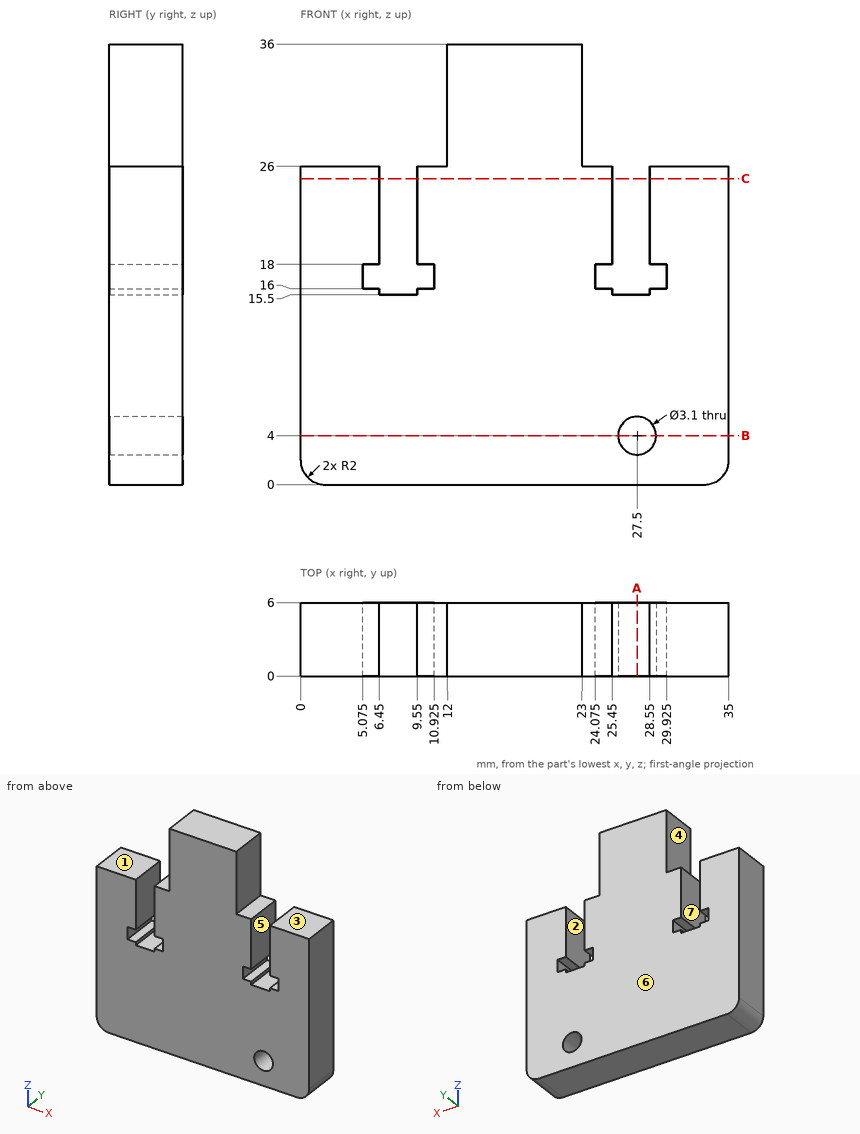
Input: dimensioned drawing with shaded views. Units: mm. Origin: part minimum x, y, z. A direction names the side the tool comes from. Round coordinates to 2 decimals unless told otherwise and drop trailing zeros. Loops run counter-clockwise (first coordinate to the right, second up) from the corner with the lowest first, then second, coordinate; pieces in that order, holes last.
1) Set-up query: the marked faces 1, 2 and 3. Return all of +Z, -Z, +X, -X, +Y, -Y with unobstructed straight access to the full face (end or side cutting, diameter ignored); none if empty.
Ans:
face 1: +Z, -X, +Y, -Y
face 2: +Z, +Y, -Y
face 3: +Z, +X, +Y, -Y
2) Section query C-C on z = 25. Return the cut outline in (x, y), plus the area to 3 significant figures.
Ans:
outline: (0, 0) - (6.45, 0) - (6.45, 6) - (0, 6) - close; (9.55, 0) - (25.45, 0) - (25.45, 6) - (9.55, 6) - close; (28.55, 0) - (35, 0) - (35, 6) - (28.55, 6) - close
area: 173 mm2
3) Pin query (flat end, axial travel): pin 1 (1.8 mm diameter, centred on y = 2, z = 30, fed in from -X); pin 2 (1.5 mm diameter, centred on x = 27, y = 3, fed in from +Z); pin 3 (0.7 mm diameter, centred on x = 23.5, y = 3, fed in from +Z). Return the tip coordinate at first contact, or that it passes through.
Ans:
pin 1: stops at x = 12
pin 2: stops at z = 15.5
pin 3: stops at z = 26
4) Pull-direction query (X, two-part tool) for the marked faces 4, 5, 6 and 7; classes: released by +X, released by -X, zero draft, split by the parting line, or undercut.
Ans:
face 4: released by -X
face 5: undercut
face 6: zero draft
face 7: undercut
5) Section query A-A on x = 27.5. Return the cut outline in (y, z), plus the area to 3 significant figures.
Ans:
outline: (0, 0) - (6, 0) - (6, 2.45) - (0, 2.45) - close; (0, 5.55) - (6, 5.55) - (6, 15.5) - (0, 15.5) - close
area: 74.4 mm2
6) Section query B-B on z = 4. Return the cut outline in (x, y).
Ans:
outline: (0, 0) - (25.95, 0) - (25.95, 6) - (0, 6) - close; (29.05, 0) - (35, 0) - (35, 6) - (29.05, 6) - close
7) Material intervals for line 1 (X direction, y = 3.45, z = 25); line 2 (Z direction, x = 29.5, y = 3.15); line 3 (X direction, y = 4.15, z = 4), sorted ascending.
Ans:
line 1: x = 0 to 6.45, 9.55 to 25.45, 28.55 to 35
line 2: z = 0 to 16, 18 to 26
line 3: x = 0 to 25.95, 29.05 to 35
